Can you work these out from the model? Positions are in its coordinate system, mm. Give positions to 0.01 mm unless a question says otherwise; leave off trailing zeros. Write each loop counter-clockwise with the first axis right and the second up, starting at its lowest first coordinate (ties: lowest second). Pieces come first, ordered by that corner, then holes.
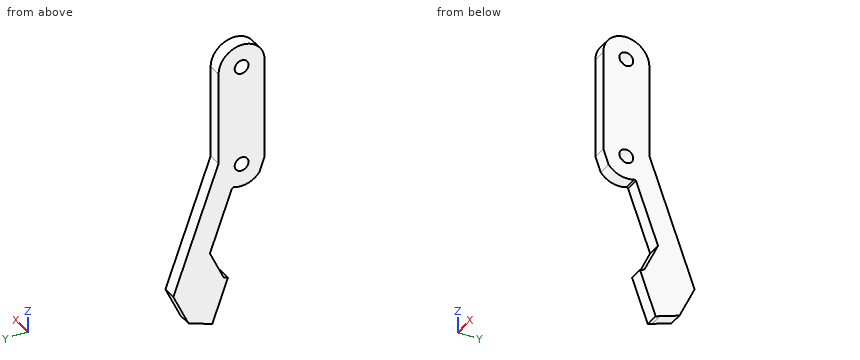
from build123d import *

# Parameters (mm, degrees)
SKETCH1_R           = 5
SKETCH1_R_2         = 1.5
BOSS_EXTRUDE1_DEPTH = 3
BOSS_EXTRUDE2_DEPTH = 3
CUT_EXTRUDE1_DEPTH  = 3
CUT_EXTRUDE2_DEPTH  = 4


with BuildPart() as part:
    # Sketch1 → Boss-Extrude1 (new body)
    with BuildSketch(Plane(origin=(0, 0, 0), x_dir=(0, 0, -1), z_dir=(1, 0, 0))):
        with Locations((5, 5)):
            Circle(SKETCH1_R)
        with Locations((5, 5)):
            Circle(SKETCH1_R_2, mode=Mode.SUBTRACT)
        with BuildLine():
            ThreePointArc((10, 5), (8.535533906, 1.464466094), (5, 0))
            Line((5, 0), (27, 0))
            ThreePointArc((27, 0), (22, 5), (27, 10))
            Line((27, 10), (5, 10))
            ThreePointArc((5, 10), (8.535533906, 8.535533906), (10, 5))
        make_face()
        with Locations((27, 5)):
            Circle(SKETCH1_R)
        with Locations((27, 5)):
            Circle(SKETCH1_R_2, mode=Mode.SUBTRACT)
    extrude(amount=BOSS_EXTRUDE1_DEPTH)

    # Sketch2 → Boss-Extrude2 (add)
    with BuildSketch(Plane(origin=(3, 0, 0), x_dir=(0, 0, -1), z_dir=(1, 0, 0))):
        with BuildLine():
            ThreePointArc((27, 10), (29.863119288, 9.099091112), (31.69447473, 6.721019177))
            Line((31.69447473, 6.721019177), (31.867747629, 7.092604107))
            Line((31.867747629, 7.092604107), (45.02344432, 11.880886114))
            Line((45.02344432, 11.880886114), (51.43200814, 8.892523726))
            Line((51.43200814, 8.892523726), (60.828934348, 12.31272516))
            Line((60.828934348, 12.31272516), (57.408732915, 21.709651368))
            Line((57.408732915, 21.709651368), (25.236730193, 10))
            Line((25.236730193, 10), (27, 10))
        make_face()
        Polygon((60.828934348, 12.31272516), (51.43200814, 8.892523726), (51.774028284, 7.952831106), (61.170954492, 11.373032539), align=None)
    extrude(amount=-BOSS_EXTRUDE2_DEPTH)

    # Sketch3 → Cut-Extrude1 (cut)
    with BuildSketch(Plane(origin=(3, 0, 0), x_dir=(0, 0, -1), z_dir=(1, 0, 0))):
        with BuildLine():
            ThreePointArc((27, 0), (28.710100717, 0.301536896), (30.213938048, 1.169777784))
            Line((30.213938048, 1.169777784), (27, 0))
        make_face()
    extrude(amount=-CUT_EXTRUDE1_DEPTH, mode=Mode.SUBTRACT)

    # Sketch4 → Cut-Extrude2 (cut, through all)
    with BuildSketch(Plane(origin=(3, 0, 0), x_dir=(0, 0, -1), z_dir=(1, 0, 0))):
        Polygon((57.408732915, 21.709651368), (52.240423501, 19.828540579), (59.289843703, 16.541341953), align=None)
    extrude(amount=-CUT_EXTRUDE2_DEPTH, mode=Mode.SUBTRACT)


solid = part.part
(1) If I drill on L1, parallel to Y at x = 2, z = -15; L2, parallel to Y at x = 1.4, z = -5; L3, parallel to Z at x = 2.55, y = 4.75, over which ranges is the centre line in solid material (lowest first)?
Returned:
L1: y = 0 to 10
L2: y = 0 to 3.5, 6.5 to 10
L3: z = -31.99 to -28.48, -25.52 to -6.48, -3.52 to -0.01
(2) Imagine slicing it at C-C, the plane z = -21.5. Write out the boundary of the cut face in (x, y).
Returned:
outline: (0, 0) - (3, 0) - (3, 10) - (0, 10) - close
(3) Imagine slicing it at B-B, the plane x = 0.7. Write out the boundary of the cut face in (y, z).
Returned:
outline: (0, -27) - (1.17, -30.21) arc R5 ccw to (6.72, -31.69) - (7.09, -31.87) - (11.88, -45.02) - (8.89, -51.43) - (7.95, -51.77) - (11.37, -61.17) - (16.54, -59.29) - (19.83, -52.24) - (10, -25.24) - (10, -5) arc R5 ccw to (0, -5) - close; hole circle Ø3 at (5, -27); hole circle Ø3 at (5, -5)
(4) Imagine slicing it at D-D, the plane y = 16. Write out the boundary of the cut face in (x, z).
Returned:
outline: (0, -59.49) - (3, -59.49) - (3, -41.72) - (0, -41.72) - close
(5) Imagine slicing it at A-A, the plane y = 5. Write out the boundary of the cut face in (x, z), plus the area to 3 significant figures.
Returned:
outline: (0, -32) - (3, -32) - (3, -28.5) - (0, -28.5) - close; (0, -25.5) - (3, -25.5) - (3, -6.5) - (0, -6.5) - close; (0, -3.5) - (3, -3.5) - (3, 0) - (0, 0) - close
area: 78.0 mm2
